from build123d import *

# Parameters (mm, degrees)
SKETCH2_W           = 145
SKETCH2_H           = 165
BOSS_EXTRUDE1_DEPTH = 4
SKETCH2_3_W         = 10
SKETCH2_3_H         = 165
CUT_EXTRUDE1_DEPTH  = 2.5
SKETCH3_R           = 0.98
CUT_EXTRUDE3_DEPTH  = 5
SKETCH5_R           = 0.98
CUT_EXTRUDE4_DEPTH  = 4


with BuildPart() as part:
    # Sketch2 → Boss-Extrude1 (new body)
    with BuildSketch(Plane(origin=(0, 0, 0), x_dir=(1, 0, 0), z_dir=(0, 1, 0))):
        Rectangle(SKETCH2_W, SKETCH2_H)
    extrude(amount=-BOSS_EXTRUDE1_DEPTH)

    # Sketch2<3> → Cut-Extrude1 (cut)
    with BuildSketch(Plane(origin=(0, 0, 0), x_dir=(1, 0, 0), z_dir=(0, 1, 0))):
        with Locations((-19.5, 0)):
            Rectangle(SKETCH2_3_W, SKETCH2_3_H)
        with Locations((-58.5, 0)):
            Rectangle(SKETCH2_3_W, SKETCH2_3_H)
        with Locations((19.5, 0)):
            Rectangle(SKETCH2_3_W, SKETCH2_3_H)
        with Locations((58.5, 0)):
            Rectangle(SKETCH2_3_W, SKETCH2_3_H)
    extrude(amount=-CUT_EXTRUDE1_DEPTH, mode=Mode.SUBTRACT)

    # Sketch3 → Cut-Extrude3 (cut)
    with BuildSketch(Plane.XZ.offset(4)):
        with Locations((-70, 80)):
            Circle(SKETCH3_R)
        with Locations((70, 80)):
            Circle(SKETCH3_R)
        with Locations((70, -80)):
            Circle(SKETCH3_R)
        with Locations((-70, -80)):
            Circle(SKETCH3_R)
    extrude(amount=-CUT_EXTRUDE3_DEPTH, mode=Mode.SUBTRACT)

    # Sketch5 → Cut-Extrude4 (cut)
    with BuildSketch(Plane(origin=(0, -4, 0), x_dir=(1, 0, 0), z_dir=(0, 1, 0))):
        with Locations((-35.438735521, -29.971809351)):
            Circle(SKETCH5_R)
        with Locations((38.831264479, -29.971809351)):
            Circle(SKETCH5_R)
        with Locations((38.831264479, -65.811809351)):
            Circle(SKETCH5_R)
        with Locations((-35.438735521, -65.811809351)):
            Circle(SKETCH5_R)
    extrude(amount=CUT_EXTRUDE4_DEPTH, mode=Mode.SUBTRACT)


solid = part.part
The model under review builds one solid part; all positions refer to its coordinate system, in mm. A direction names the side the tool comes from. Round coordinates to 2 decimals unless told otherwise and drop trailing zeros. Write each loop counter-clockwise with the first axis right and the second up, starting at its lowest first coordinate (ties: lowest second). Pieces come first, ordered by that corner, then holes. Notation, with made-up numbers: M 41,41.25 L 57,41.25 A23 cw 57,79.25 Z; hole C -22.5,-14 d11. An arc over 180 degrees is marked long. Answer as CSV lines item,"result". Start each with the question number.
Q1. Consider section A-A, the plane y = -1. State how many separate pieces and enclosed holes the cut face has, then the cut area to 3 significant figures.
Q2. The part is to be moulded in two halves that separate along X. For faces 1 (the face through (-72.5, -2, 1)), 2 (the face through (19, -2.5, -1)), 3 (the face through (-1, -2, -82.5)), say which applies: +X half, -X half, draft (parallel to the pull), parting line (faces both ways), or undercut.
Q3. Wall thickness on line 1 along Z through (x, y) = (-70, -1.6); line 2 along X through (y, z) = (-1.6, 39); line 3 along X through (y, z) = (-3, -80): over which ranges is each line inside the solid? List them lowest first.
Q4. Clearance check with flat-ended pins moving along their axes: P1, Ø1.2, axis at x = -35.44, z = 29.97, coming from the +Y side; P2, Ø5, axis at x = -47, z = -48, coming from the +Y side; P3, Ø3, axis at x = 59, z = 8, coming from the +Y side. State where each tip first meets the part, or that it passes through.
Q5. Tool access review of faces 4 (the face through (58, -2.5, -1)), 5 (the face through (-68, 0, -1)): name each direction out of +Z, -Z, +X, -X, +Y, -Y from which nothing blocks a thin tool from reaching the whole face with its end or side.
Q6. Consider section B-B, the plane z = -38.5. Give the boundary of the cut face in (x, y), then the cut area to 3 significant figures.
Result set:
1,separate pieces,"5"
1,enclosed holes,"8"
1,area,"17,300 mm²"
2,face 1,"-X half"
2,face 2,"undercut"
2,face 3,"draft"
3,line 1,"z = -82.5 to -80.98, -79.02 to 79.02, 80.98 to 82.5"
3,line 2,"x = -72.5 to -63.5, -53.5 to -24.5, -14.5 to 14.5, 24.5 to 53.5, 63.5 to 72.5"
3,line 3,"x = -72.5 to -70.98, -69.02 to 69.02, 70.98 to 72.5"
4,P1,"passes through"
4,P2,"stops at y = 0"
4,P3,"stops at y = -2.5"
5,face 4,"+Z, -Z, +Y"
5,face 5,"+Z, -Z, +X, -X, +Y"
6,outline,"M -72.5,-4 L 72.5,-4 L 72.5,0 L 63.5,0 L 63.5,-2.5 L 53.5,-2.5 L 53.5,0 L 24.5,0 L 24.5,-2.5 L 14.5,-2.5 L 14.5,0 L -14.5,0 L -14.5,-2.5 L -24.5,-2.5 L -24.5,0 L -53.5,0 L -53.5,-2.5 L -63.5,-2.5 L -63.5,0 L -72.5,0 Z"
6,area,"480 mm²"
